Build history of the part. All positions in model axes, mm. A direction names the side the tool comes from. Round coordinates to 2 decimals unless told otherwise and drop trailing zeros. Write each loop counter-clockwise with the first axis right and the second up, starting at its lowest first coordinate (ties: lowest second). Pieces come first, ordered by that corner, then holes. Notation, with made-up numbers: (-25.75, -27.75) -> (21.25, -27.75) arc R29 ccw to (21.25, -0.75) -> close; hole circle Ø10 at (68.5, 16.5). An arc over 180 degrees is marked (long way). Answer as CSV lines item,"result".
from build123d import *

# Parameters (mm, degrees)
SKETCH_1_R          = 2.5
EXTRUDE_1_DEPTH     = 180
SKETCH_2_R          = 82.250528809
CUT_EXTRUDE_1_DEPTH = 10
SKETCH_3_R          = 47.359827943
CUT_EXTRUDE_2_DEPTH = 200
SKETCH_4_R          = 50.055938799
CUT_EXTRUDE_3_DEPTH = 30


with BuildPart() as part:
    # 草图1 → 凸台-拉伸1 (new, symmetric)
    with BuildSketch(Plane(origin=(0, 0, 0), x_dir=(1, 0, 0), z_dir=(0, 1, 0))):
        Polygon((-15, -3.15), (-12.5, -3.15), (-12.5, -5.15), (-7, -5.15), (-7, -3.15), (-4.5, -3.15), (-4.5, 3.15), (-7, 3.15), (-7, 5.15), (-12.5, 5.15), (-12.5, 3.15), (-15, 3.15), (-15, 15), (-3.15, 15), (-3.15, 12.5), (-5.15, 12.5), (-5.15, 7), (-3.15, 7), (-3.15, 4.5), (3.15, 4.5), (3.15, 7), (5.15, 7), (5.15, 12.5), (3.15, 12.5), (3.15, 15), (15, 15), (15, 3.15), (12.5, 3.15), (12.5, 5.15), (7, 5.15), (7, 3.15), (4.5, 3.15), (4.5, -3.15), (7, -3.15), (7, -5.15), (12.5, -5.15), (12.5, -3.15), (15, -3.15), (15, -15), (3.15, -15), (3.15, -12.5), (5.15, -12.5), (5.15, -7), (3.15, -7), (3.15, -4.5), (-3.15, -4.5), (-3.15, -7), (-5.15, -7), (-5.15, -12.5), (-3.15, -12.5), (-3.15, -15), (-15, -15), align=None)
        with Locations(Location((-9.75, -9.75, 0), (0, 0, 90))):
            Circle(SKETCH_1_R, mode=Mode.SUBTRACT)
        with Locations(Location((-9.75, 9.75, 0), (0, 0, 90))):
            Circle(SKETCH_1_R, mode=Mode.SUBTRACT)
        with Locations(Location((9.75, 9.75, 0), (0, 0, 90))):
            Circle(SKETCH_1_R, mode=Mode.SUBTRACT)
        with Locations(Location((9.75, -9.75, 0), (0, 0, 90))):
            Circle(SKETCH_1_R, mode=Mode.SUBTRACT)
    extrude(amount=EXTRUDE_1_DEPTH, both=True)

    # 草图2 → 切除-拉伸1 (cut)
    with BuildSketch(Plane(origin=(0, 180, 0), x_dir=(1, 0, 0), z_dir=(0, 1, 0))):
        Circle(SKETCH_2_R)
    extrude(amount=-CUT_EXTRUDE_1_DEPTH, mode=Mode.SUBTRACT)

    # 草图3 → 切除-拉伸2 (cut)
    with BuildSketch(Plane.XZ.offset(180)):
        with Locations((0.216432031, -1.772037256)):
            Circle(SKETCH_3_R)
    extrude(amount=-CUT_EXTRUDE_2_DEPTH, mode=Mode.SUBTRACT)

    # 草图4 → 切除-拉伸3 (cut)
    with BuildSketch(Plane.XZ.offset(-20)):
        with Locations((-1.287426062, -1.543634952)):
            Circle(SKETCH_4_R)
    extrude(amount=-CUT_EXTRUDE_3_DEPTH, mode=Mode.SUBTRACT)


solid = part.part
1. Cut at C-C, the plane y = 118. Count the separate pieces of the cut face and the enclosed holes in it, then the cut area to 3 significant figures.
Results found:
separate pieces,"1"
enclosed holes,"4"
area,"469 mm2"
2. Cut at B-B, the plane z = -9.75. Write the cut outline in (x, y), then the cut area to 3 significant figures.
Results found:
outline,"(-15, 50) -> (-12.25, 50) -> (-12.25, 170) -> (-15, 170) -> close; (-7.25, 50) -> (-5.15, 50) -> (-5.15, 170) -> (-7.25, 170) -> close; (5.15, 50) -> (7.25, 50) -> (7.25, 170) -> (5.15, 170) -> close; (12.25, 50) -> (15, 50) -> (15, 170) -> (12.25, 170) -> close"
area,"1,160 mm2"
3. Drop flat-ended pins along their axis: pin 1 Ø3 at (y, z) = (71, 1) entering from +X; pin 2 Ø5 at (x, y) = (1, 89) entering from +Z. Give the stop position or say it passes through.
Results found:
pin 1,"stops at x = 4.5"
pin 2,"stops at z = 15"
4. Probe line 1 along Z through (x, y) = (10, 108); line 2 along X through (y, z) = (82, 9.75); line 3 along X through (y, z) = (67, -4). List the from-to ranges inside material, lowest first.
Results found:
line 1,"z = -15 to -12.24, -7.26 to -5.15, 5.15 to 7.26, 12.24 to 15"
line 2,"x = -15 to -12.25, -7.25 to -5.15, 5.15 to 7.25, 12.25 to 15"
line 3,"x = -15 to -12.5, -7 to 7, 12.5 to 15"
5. Which spindle directions (+Z, -Z, +X, -X, +Y, -Y) get a long thin tool onto all of the face, cutting with end or side? Do faces 1 (the flat face through (-6, 111, -3.15)), 2 (the flat face through (14, 111, 3.15)), 3 (the flat face through (-4, 111, 7)), 4 (the flat face through (3.15, 111, 14)), 5 (the flat face through (3.15, 111, -14)). Say none if no direction does.
Results found:
face 1,"-X, +Y, -Y"
face 2,"+X, +Y, -Y"
face 3,"+Y, -Y"
face 4,"+Z, +Y, -Y"
face 5,"-Z, +Y, -Y"
6. Cut at D-D, the plane z = 0. Write the cut outline in (x, y), then the cut area to 3 significant figures.
Results found:
outline,"(-4.5, 50) -> (4.5, 50) -> (4.5, 170) -> (-4.5, 170) -> close"
area,"1,080 mm2"
7. Mould opens along Z. For faces 6 (the cylindrical face through (12.19, 109.16, 10.29)), 7 (the flat face through (-3.15, 111, 14)), 8 (the flat face through (0, 111, 4.5)) say: +Z half, -Z half, draft (parallel to the pull), parting line (faces both ways), or undercut.
Results found:
face 6,"undercut"
face 7,"draft"
face 8,"+Z half"
8. Cut at A-A, the plane x = 9.75. Write the cut outline in (y, z), then the cut area to 3 significant figures.
Results found:
outline,"(50, -15) -> (170, -15) -> (170, -12.25) -> (50, -12.25) -> close; (50, -7.25) -> (170, -7.25) -> (170, -5.15) -> (50, -5.15) -> close; (50, 5.15) -> (170, 5.15) -> (170, 7.25) -> (50, 7.25) -> close; (50, 12.25) -> (170, 12.25) -> (170, 15) -> (50, 15) -> close"
area,"1,160 mm2"
